Geometry check sheet. Reference: the model listing, model coordinates, mm. A direction names the side the tool comes from. Give positions to 0.01 mm unless a question says otherwise; leave off trailing zeros. Order: outer loops, then holes, each group sorted by start corner. A loop starts at its lowest first (then second) coordinate and runs counter-clockwise, first axis right, second up. Notation, with made-up numbers: M -3.5,27.25 L 34.5,27.25 A26 cw 34.5,57.25 Z; hole C 60,2 d5. An arc over 180 degrees is marked long. Answer as a JSON object with one key per item and string values. Group by question number.
from build123d import *

# Parameters (mm, degrees)
SKETCH1_R           = 4.25
SKETCH1_R_2         = 1.5
BOSS_EXTRUDE1_DEPTH = 2
SKETCH2_R           = 9.5
BOSS_EXTRUDE2_DEPTH = 6


with BuildPart() as part:
    # Sketch1 → Boss-Extrude1 (new body)
    with BuildSketch(Plane(origin=(0, 0, 0), x_dir=(1, 0, 0), z_dir=(0, 1, 0))):
        Polygon((-15, 11), (-11, 15), (11, 15), (15, 11), (15, -11), (11, -15), (-11, -15), (-15, -11), align=None)
        with Locations(Location((0, 0, 0), (0, 0, 270))):
            Circle(SKETCH1_R, mode=Mode.SUBTRACT)
        with Locations(Location((-10.878679656, -10.878679656, 0), (0, 0, 270))):
            Circle(SKETCH1_R_2, mode=Mode.SUBTRACT)
        with Locations(Location((-10.878679656, 10.878679656, 0), (0, 0, 270))):
            Circle(SKETCH1_R_2, mode=Mode.SUBTRACT)
        with Locations(Location((10.878679656, 10.878679656, 0), (0, 0, 270))):
            Circle(SKETCH1_R_2, mode=Mode.SUBTRACT)
        with Locations(Location((10.878679656, -10.878679656, 0), (0, 0, 270))):
            Circle(SKETCH1_R_2, mode=Mode.SUBTRACT)
    extrude(amount=BOSS_EXTRUDE1_DEPTH)

    # Sketch2 → Boss-Extrude2 (add)
    with BuildSketch(Plane(origin=(0, 2, 0), x_dir=(1, 0, 0), z_dir=(0, 1, 0))):
        with Locations(Location((0, 0, 0), (0, 0, 90))):
            Circle(SKETCH2_R)
        Polygon((7.505553499, 0), (3.75277675, 6.5), (-3.75277675, 6.5), (-7.505553499, 0), (-3.75277675, -6.5), (3.75277675, -6.5), align=None, mode=Mode.SUBTRACT)
    extrude(amount=BOSS_EXTRUDE2_DEPTH)


solid = part.part
1. Cross-section at C-C (z = -1.75). Record the cut outline in (x, y), and give its area (3 significant figures).
2. Release check for a two-part mould opening along X. For faces 1 (the flat face through (0, 5, 6.5)), 2 (the flat face through (15, 1, 0)), 3 (the flat face through (7, 2, -7)) record: released by +X, released by -X, zero draft, split by the parting line, or undercut.
3. Access from +Z, -Z, +X, -X, +Y, -Y to the whole of each face (thin tool, end or side, straight path). Record for faces 4 (the flat face through (-15, 1, 0)), 5 (the flat face through (5.66, 4.96, -3.2)).
4. Cross-section at B-B (y = 5.25). Record the cut outline in (x, z), and give its area (3 significant figures).
5. Cross-section at A-A (x = 0). Record the cut outline in (y, z).
6. Cross-section at D-D (z = -12). Record the cut outline in (x, y) (3 decimals).
7. Depth check by flat-ended pin: pin 1 (14.5 mm diameter, centred on x = 3, z = -2, fed in from +Y). Enter the tip coordinate at first touch or a pass-through.
8. Thickness scan on line 1 along Z through (x, y) = (1.5, 3.25); line 2 along Y through (x, z) = (6.75, -12); line 3 along X through (y, z) = (0.8, 0). Record the ranges inside material, lowest first. Write a range as [from, to].
Report:
{
 "1": {"outline": "M -15,0 L -3.87,0 L -3.87,2 L -6.5,2 L -6.5,8 L -9.34,8 L -9.34,2 L -15,2 Z; M 3.87,0 L 15,0 L 15,2 L 9.34,2 L 9.34,8 L 6.5,8 L 6.5,2 L 3.87,2 Z", "area": "78.6 mm2"},
 "2": {"face 1": "undercut", "face 2": "released by +X", "face 3": "zero draft"},
 "3": {"face 4": "+Z, -Z, -X, +Y, -Y", "face 5": "+Y"},
 "4": {"outline": "C 0,0 d19; hole M -7.51,0 L -3.75,-6.5 L 3.75,-6.5 L 7.51,0 L 3.75,6.5 L -3.75,6.5 Z", "area": "137 mm2"},
 "5": {"outline": "M 0,-15 L 2,-15 L 2,-9.5 L 8,-9.5 L 8,-6.5 L 2,-6.5 L 2,-4.25 L 0,-4.25 Z; M 0,4.25 L 2,4.25 L 2,6.5 L 8,6.5 L 8,9.5 L 2,9.5 L 2,15 L 0,15 Z"},
 "6": {"outline": "M -14,0 L -11.875,0 L -11.875,2 L -14,2 Z; M -9.882,0 L 9.882,0 L 9.882,2 L -9.882,2 Z; M 11.875,0 L 14,0 L 14,2 L 11.875,2 Z"},
 "7": {"pin 1": "stops at y = 8"},
 "8": {"line 1": "z = [-9.38, -6.5], [6.5, 9.38]", "line 2": "y = [0, 2]", "line 3": "x = [-15, -4.25], [4.25, 15]"}
}
